```python
from build123d import *

# Parameters (mm, degrees)
SKETCH1_W           = 203.2
SKETCH1_H           = 152.4
SKETCH1_R           = 3.175
BOSS_EXTRUDE1_DEPTH = 12.7


with BuildPart() as part:
    # Sketch1 → Boss-Extrude1 (new body)
    with BuildSketch(Plane(origin=(0, 0, 0), x_dir=(0, 0, -1), z_dir=(1, 0, 0))):
        Rectangle(SKETCH1_W, SKETCH1_H)
        with Locations((-15.875, -63.5)):
            Circle(SKETCH1_R, mode=Mode.SUBTRACT)
        with Locations((-15.875, 0)):
            Circle(SKETCH1_R, mode=Mode.SUBTRACT)
        with Locations((92.075, 0)):
            Circle(SKETCH1_R, mode=Mode.SUBTRACT)
        with Locations((92.075, -63.5)):
            Circle(SKETCH1_R, mode=Mode.SUBTRACT)
        with Locations((-92.075, -63.5)):
            Circle(SKETCH1_R, mode=Mode.SUBTRACT)
        with Locations((-92.075, 0)):
            Circle(SKETCH1_R, mode=Mode.SUBTRACT)
        with Locations((92.075, 57.15)):
            Circle(SKETCH1_R, mode=Mode.SUBTRACT)
        with Locations((-15.875, 57.15)):
            Circle(SKETCH1_R, mode=Mode.SUBTRACT)
        with Locations((-92.075, 57.15)):
            Circle(SKETCH1_R, mode=Mode.SUBTRACT)
        with BuildLine():
            ThreePointArc((17.261210647, 30.43), (18.461210647, 29.23), (17.261210647, 28.03))
            Line((17.261210647, 28.03), (14.661210647, 28.03))
            ThreePointArc((14.661210647, 28.03), (13.461210647, 29.23), (14.661210647, 30.43))
            Line((14.661210647, 30.43), (17.261210647, 30.43))
        make_face(mode=Mode.SUBTRACT)
        with BuildLine():
            Line((41.801210647, 28.03), (39.201210647, 28.03))
            ThreePointArc((39.201210647, 28.03), (38.001210647, 29.23), (39.201210647, 30.43))
            Line((39.201210647, 30.43), (41.801210647, 30.43))
            ThreePointArc((41.801210647, 30.43), (43.001210647, 29.23), (41.801210647, 28.03))
        make_face(mode=Mode.SUBTRACT)
        with BuildLine():
            Line((14.661210647, 48.17), (17.261210647, 48.17))
            ThreePointArc((17.261210647, 48.17), (18.461210647, 46.97), (17.261210647, 45.77))
            Line((17.261210647, 45.77), (14.661210647, 45.77))
            ThreePointArc((14.661210647, 45.77), (13.461210647, 46.97), (14.661210647, 48.17))
        make_face(mode=Mode.SUBTRACT)
        with BuildLine():
            ThreePointArc((41.801210647, 48.17), (43.001210647, 46.97), (41.801210647, 45.77))
            Line((41.801210647, 45.77), (39.201210647, 45.77))
            ThreePointArc((39.201210647, 45.77), (38.001210647, 46.97), (39.201210647, 48.17))
            Line((39.201210647, 48.17), (41.801210647, 48.17))
        make_face(mode=Mode.SUBTRACT)
    extrude(amount=BOSS_EXTRUDE1_DEPTH)


solid = part.part
```
Part model, mm, in its own coordinate system. Coordinates: 2 decimals unless noted, no trailing zeros. Order: outer loops, then holes, each group sorted by start corner. A loop starts at its lowest first (then second) coordinate and runs counter-clockwise, first axis right, second up. Notation, with made-up numbers: (7, 77.25) -> (55, 77.25) arc R20 ccw to (55, 94.25) -> close; hole circle Ø6 at (13.25, -22.75). An arc over 180 degrees is marked (long way). Put each result on its own line as item: value. Start each with the question number.
(1) Probe line 1 along Y through (x, z) = (11.25, -39.5). List the from-to ranges inside material, lowest first. Write a range as [from, to].
(2) Mould opens along Y. For faces 1 (the face through (0, 1, 1)), 2 (the face through (6, -76.2, 1)), 3 (the face through (6.261, 0.954, 12.847)) say: pulls with the +Y half, pulls with the -Y half, needs draft (parallel to the pull), parting line crosses it, or undercut.
(3) Band-saw the part on A-A (y = 0). Give the cut face in (x, z), then the cut area to 3 significant figures.
Determined:
1. line 1: y = [-76.2, 28.03], [30.43, 45.77], [48.17, 76.2]
2. face 1: needs draft
2. face 2: pulls with the -Y half
2. face 3: undercut
3. outline: (0, -101.6) -> (12.7, -101.6) -> (12.7, -95.25) -> (0, -95.25) -> close; (0, -88.9) -> (12.7, -88.9) -> (12.7, 12.7) -> (0, 12.7) -> close; (0, 19.05) -> (12.7, 19.05) -> (12.7, 88.9) -> (0, 88.9) -> close; (0, 95.25) -> (12.7, 95.25) -> (12.7, 101.6) -> (0, 101.6) -> close
3. area: 2,340 mm²
